Verification items for this drawing (mm, ordinates from the low corner). A direction names the side the tool comes from. Coordinates: 2 decimals unless noted, no trailing zeros. Write each loop counter-clockwise with the first axis right and the second up, starting at its lowest first coordinate (ties: lowest second). Pieces come first, ordered by that corner, then holes. Notation, with made-up numbers: (32.5, 46) -> (36.5, 46) arc R6 cw to (36.5, 53) -> close; hole circle Ø10 at (-35, -34). An arc over 180 degrees is marked (long way). Put each result on its own line as item: value. Start each with the question number.
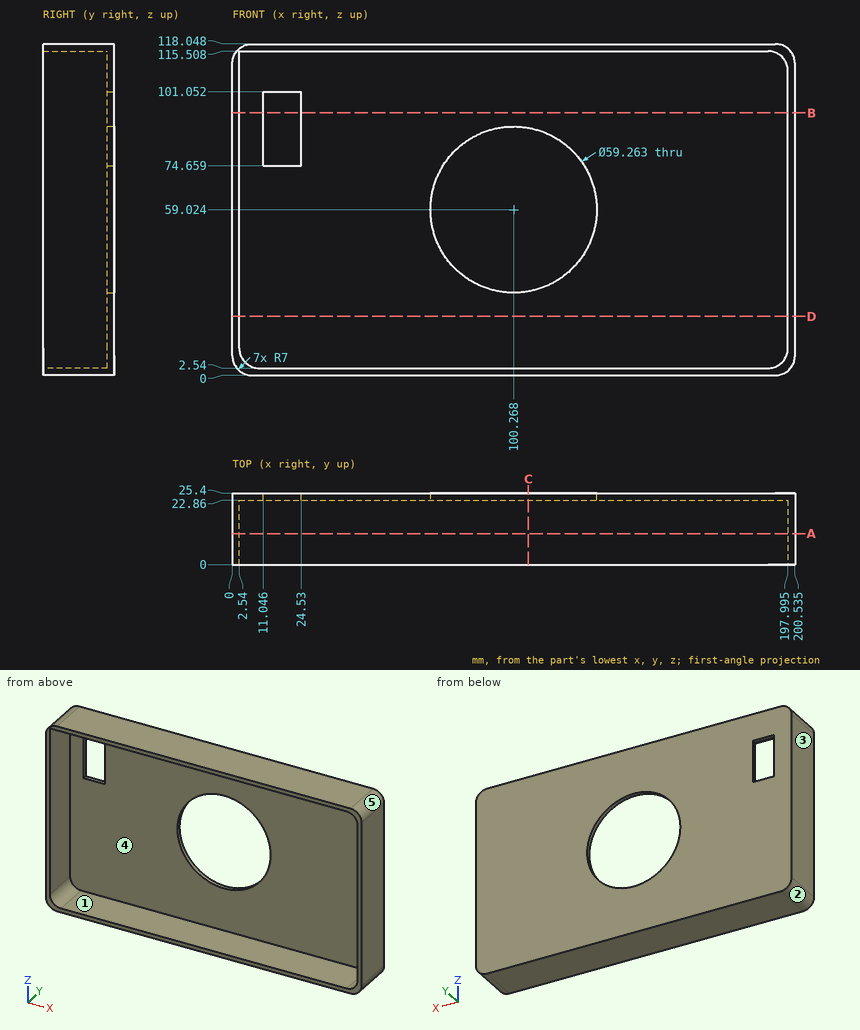
Item 1: Mould release check, pull along Z, two halves, no side actions. Record for the marked faces 1, 2 and 3: released by +Z, released by -Z, zero draft, split by the parting line, or undercut.
Item 2: Access from +Z, -Z, +X, -X, +Y, -Y to the whole of each face (thin tool, end or side, straight path). Record for the marked faces 4 and 5.
Item 3: Go/stop test with flat-tipped pins: P1, Ø11.5, axis at x = 85.5, y = 9, coming from the -Z side; P2, Ø8, axis at x = 71, z = 75.5, coming from the -Y side. Record where each tip stops, or that it passes through.
Item 4: Section check A-A, the plane y = 11. Enter the section's corners in (x, z) (1 decimal).
Item 5: Section check D-D, the plane z = 21. Enter the section's corners in (x, y) (1 decimal).
Item 6: Scan lines: line 1 along Z through (x, y) = (35.5, 16.5); line 2 along X through (y, z) = (9.25, 84.5) (1 decimal); line 3 along Y through (x, z) = (102.5, 90.5). Record each from-to range of solid material in increasing order. Write a range as [from, to].
Item 7: Section check B-B, the plane z = 93.5. Enter the section's corners in (x, y) (1 decimal).
Item 8: Section check C-C, the plane x = 105.5. Enter the section's corners in (y, z).
From the geometry:
1. face 1: undercut
1. face 2: released by -Z
1. face 3: zero draft
2. face 4: -Y
2. face 5: +Z, +X, +Y, -Y
3. P1: z = 0
3. P2: y = 22.86
4. outline: (0, 7) arc R7 ccw to (7, 0) -> (193.5, 0) arc R7 ccw to (200.5, 7) -> (200.5, 111) arc R7 ccw to (193.5, 118) -> (7, 118) arc R7 ccw to (0, 111) -> close; hole (2.5, 9.5) arc R7 ccw to (9.5, 2.5) -> (191, 2.5) arc R7 ccw to (198, 9.5) -> (198, 108.5) arc R7 ccw to (191, 115.5) -> (2.5, 115.5) -> close
5. outline: (0, 0) -> (2.5, 0) -> (2.5, 22.9) -> (198, 22.9) -> (198, 0) -> (200.5, 0) -> (200.5, 25.4) -> (0, 25.4) -> close
6. line 1: [0, 2.54], [115.51, 118.05]
6. line 2: [0, 2.5], [198, 200.5]
6. line 3: [22.86, 25.4]
7. outline: (0, 0) -> (2.5, 0) -> (2.5, 22.9) -> (11, 22.9) -> (11, 25.4) -> (0, 25.4) -> close; (24.5, 22.9) -> (198, 22.9) -> (198, 0) -> (200.5, 0) -> (200.5, 25.4) -> (24.5, 25.4) -> close
8. outline: (0, 0) -> (25.4, 0) -> (25.4, 29.86) -> (22.86, 29.86) -> (22.86, 2.54) -> (0, 2.54) -> close; (0, 115.51) -> (22.86, 115.51) -> (22.86, 88.19) -> (25.4, 88.19) -> (25.4, 118.05) -> (0, 118.05) -> close
